```python
from build123d import *

# Parameters (mm, degrees)
SKETCH1_R           = 1.7
BOSS_EXTRUDE1_DEPTH = 5
SKETCH3_R           = 5
CUT_EXTRUDE1_DEPTH  = 4
CHAMFER1_SIZE       = 0.3


with BuildPart() as part:
    # Sketch1 → Boss-Extrude1 (new body)
    with BuildSketch(Plane.XY):
        with BuildLine():
            Line((-16.6225, -21.2525), (-16.6225, 21.2525))
            ThreePointArc((-16.6225, 21.2525), (0, 37.875), (16.6225, 21.2525))
            Line((16.6225, 21.2525), (16.6225, -21.2525))
            ThreePointArc((16.6225, -21.2525), (0, -37.875), (-16.6225, -21.2525))
        make_face()
        with Locations((0, 26.5125)):
            Circle(SKETCH1_R, mode=Mode.SUBTRACT)
        with Locations((0, -26.5125)):
            Circle(SKETCH1_R, mode=Mode.SUBTRACT)
    extrude(amount=BOSS_EXTRUDE1_DEPTH)

    # Sketch3 → Cut-Extrude1 (cut)
    with BuildSketch(Plane.XY.offset(5)):
        with Locations((0, 26.5125)):
            Circle(SKETCH3_R)
        with Locations((0, -26.5125)):
            Circle(SKETCH3_R)
    extrude(amount=-CUT_EXTRUDE1_DEPTH, mode=Mode.SUBTRACT)

    # Sketch2 → Cut-Revolve1 (revolve, cut)
    with BuildSketch(Plane(origin=(0, 0, 0), x_dir=(0, 0, -1), z_dir=(1, 0, 0)), mode=Mode.PRIVATE) as cut_revolve1_sk:
        Polygon((-5, 5.3025), (0, 5.3025), (0, 2.3025), (-1.3, 3.6025), (-5, 3.6025), align=None)
    revolve(cut_revolve1_sk.sketch.rotate(Axis((0, 5.3025, 13.61294397), (0, 0, -1)), 270), axis=Axis((0, 5.3025, 13.61294397), (0, 0, -1)), mode=Mode.SUBTRACT)

    # Chamfer1
    chamfer1_edges = [part.edges().sort_by_distance(p)[0] for p in [
        (-5, 26.5125, 5),
        (-5, -26.5125, 5),
    ]]
    chamfer(chamfer1_edges, length=CHAMFER1_SIZE)


solid = part.part
```
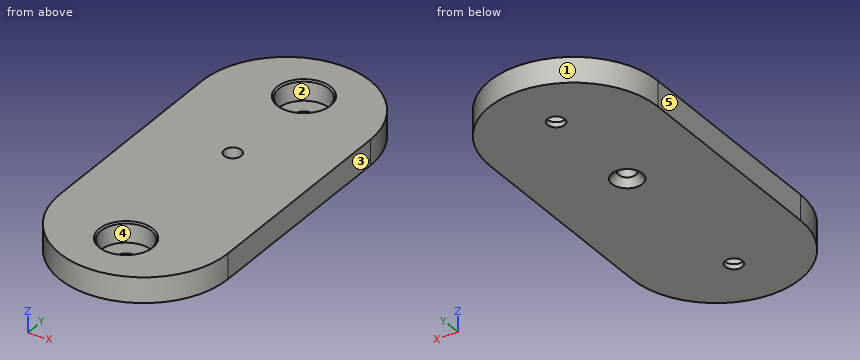
Geometry check sheet. Reference: the model listing, model coordinates, mm. Face numbers are marked on the shaded views. A direction names the side the tool comes from. Give positions to 0.01 mm unless a question says otherwise; leave off trailing zeros. Write each loop counter-clockwise with the first axis right and the second up, starting at its lowest first coordinate (ties: lowest second). Pieces come first, ordered by that corner, then holes.
1) Section check D-D, the plane x = 14. Record the boundary of the cut face in (y, z).
2) Access from +Z, -Z, +X, -X, +Y, -Y to the whole of each face (thin tool, end or side, straight path). Record for the marked faces 4 and 5.
3) Section check A-A, the plane x = 0. State how many separate pieces and enclosed holes the cut face has, and give its area (3 significant figures).
4) Release check for a two-part mould opening along X. For the marked faces 1, 2 and 3 record: pulls with the +X half, pulls with the -X half, needs draft (parallel to the pull), parting line crosses it, or undercut.
5) Section check C-C, the plane x = 6.5. Record the boundary of the cut face in (y, z), and give its area (3 significant figures).
6) Material ranges on L1, parallel to Y at x = 0, z = 2.3 (1 decimal); L2, parallel to Y at x = -2, z = 1.8; L3, parallel to Y at x = 0, z = 0.3 (1 decimal), recorded low to high.
7) Gauge pin test, flat ends, axial feed: pin 1 (1 mm diameter, centred on x = -3, z = 3.5, fed in from -Y); pin 2 (2 mm diameter, centred on x = 0, y = 5.3, fed in from +Z); pin 3 (8 mm diameter, centred on x = 0, y = -26.51, fed in from +Z). Record the tip position at first contact, or that the pin passes through.
8) Section check B-B, the plane z = 2.2. Record the boundary of the cut face in (x, y) (1 decimal).
Computed:
1. outline: (-30.21, 0) - (30.21, 0) - (30.21, 5) - (-30.21, 5) - close
2. face 4: +Z
2. face 5: +Z, -Z, -X, +Y, -Y
3. separate pieces: 4
3. enclosed holes: 0
3. area: 273 mm2
4. face 1: parting line crosses it
4. face 2: undercut
4. face 3: pulls with the +X half
5. outline: (-36.55, 0) - (36.55, 0) - (36.55, 5) - (-36.55, 5) - close
5. area: 366 mm2
6. L1: y = -37.9 to -31.5, -21.5 to 3.6, 7 to 21.5, 31.5 to 37.9
6. L2: y = -37.75 to -31.1, -21.93 to 21.93, 31.1 to 37.75
6. L3: y = -37.9 to -28.2, -24.8 to 2.6, 8 to 24.8, 28.2 to 37.9
7. pin 1: stops at y = -37.69
7. pin 2: passes through
7. pin 3: stops at z = 1
8. outline: (-16.6, -21.3) arc R16.6 ccw to (16.6, -21.3) - (16.6, 21.3) arc R16.6 ccw to (-16.6, 21.3) - close; hole circle Ø10 at (0, -26.5); hole circle Ø10 at (0, 26.5); hole circle Ø3.4 at (0, 5.3)
